Here's how the part is built. I have some questions about the finished solid (model axes, mm). A direction names the side the tool comes from. Round coordinates to 2 decimals unless told otherwise and drop trailing zeros. Write each loop counter-clockwise with the first axis right and the second up, starting at its lowest first coordinate (ties: lowest second). Pieces come first, ordered by that corner, then holes. Notation, with made-up numbers: (-22, 2.5) - (16, 2.5) arc R34 ccw to (16, 36.5) - close; hole circle Ø8 at (-3, -16). An arc over 180 degrees is marked (long way). Write item = value, one per line. Start each with the question number.
Item 1: If we section it at C-C (x = 1.5): Please give me the cut outline in (y, z).
Item 2: If I drill on line 1 along X through (y, z) = (1.25, 1.5); line 2 along X through (y, z) = (0.5, 9), over which ranges is the centre line in solid material (lowest first)? Write a range as [from, to].
Item 3: If we section it at A-A (z = 9.5): Please give me the cut outline in (x, y), and give its area (3 significant figures).
Item 4: Which directions (+Z, -Z, +X, -X, +Y, -Y) give clear straight access to the entire face, cutting with the end or side of a thin tool? Please do faces 1 (the face through (0.2, -2, 9)), 2 (the face through (-0.2, -2, 2)), 3 (the face through (-2, 0.2, 2)).
Item 5: If we section it at B-B (y = -2): Please give me the cut outline in (x, z), and give its area (3 significant figures).
Item 6: For P1, Ø1.8, axis at x = 2, z = 2, coming from the +Y side; P2, Ø1.5, axis at x = 2, y = 1, coming from the -Z side; P3, Ø1.1, axis at y = -3, z = 2, coming from the +X side; P4, Ø0.9, axis at y = 2, z = 10, coming from the -X side, each with a flat end and sliding along its axis, tell me the tip position at first contact or that it passes through.
Item 7: Thinking about a two-plate mould opening in Z: for faces 4 (the face through (0.2, -2, 2)), 5 (the face through (-2.313, 0.003, 14.391)), which applies, pulls with the +Z half, pulls with the -Z half, needs draft (parallel to the pull), parting line crosses it, or undercut?
```python
from build123d import *

# Parameters (mm, degrees)
F3_DEPTH = 0.2
F4_COUNT = 4


# Not quite as in the source:
# - a feature names something its author has since deleted; it is built from what else it names


with BuildPart() as f1:
    # F0 (on Front) → F1 (revolve)
    with BuildSketch(Plane.XZ):
        with BuildLine():
            Line((0, 24.5833333333), (0, 0))
            Line((0, 0), (0.6944444444, 0))
            Line((0.6944444444, 0), (0.6944444444, 0.2777777778))
            Line((0.6944444444, 0.2777777778), (0.9097222222, 0.625))
            Line((0.9097222222, 0.625), (0.9097222222, 20.8333333333))
            ThreePointArc((0.9097222222, 20.8333333333), (0.6790405117, 22.7627175953), (0, 24.5833333333))
        make_face()
    revolve(axis=Axis((0, 0, 12.2916666667), (0, 0, 1)))

    # F2 (on Front) → F3 (join, symmetric)
    with BuildSketch(Plane.XZ):
        with BuildLine():
            Line((0, 0.625), (0, 0.5555555556))
            Line((0, 0.5555555556), (2.7430555556, 0.5555555556))
            Line((2.7430555556, 0.5555555556), (2.7430555556, 1.1111111111))
            Line((2.7430555556, 1.1111111111), (3.8194444444, 1.1111111111))
            Line((3.8194444444, 1.1111111111), (3.3333333333, 2.7777777778))
            Line((3.3333333333, 2.7777777778), (0.8, 2.7777777778))
            Line((0.8, 2.7777777778), (0.8, 2.9458333333))
            Line((0.8, 2.9458333333), (1.1180555556, 3.2638888889))
            Line((1.1180555556, 3.2638888889), (1.1180555556, 4.1666666667))
            Line((1.1180555556, 4.1666666667), (2.7430555556, 4.1666666667))
            Line((2.7430555556, 4.1666666667), (2.7430555556, 12.9166666667))
            ThreePointArc((2.7430555556, 12.9166666667), (2.3012216629, 14.4095607148), (1.1180555556, 15.4215230609))
            Line((1.1180555556, 15.4215230609), (1.1180555556, 18.7331644265))
            Line((1.1180555556, 18.7331644265), (0, 21.8049968191))
            Line((0, 21.8049968191), (0, 0.625))
        make_face()
    extrude(amount=F3_DEPTH, both=True)

    # F4: F1 ×4 about axis
    f4_axis = Axis((0, 0, 0.625), (0, 0, 1))


with BuildPart() as f1_1:
    add(f1.part)
    for i in range(1, F4_COUNT):
        add(f1.part.rotate(f4_axis, i * 360 / F4_COUNT))


solid = f1_1.part
```
Reply:
q1.outline = (-0.2, 0.56) - (0.2, 0.56) - (0.2, 2.78) - (-0.2, 2.78) - close; (-0.2, 4.17) - (0.2, 4.17) - (0.2, 15.21) - (-0.2, 15.21) - close
q2.line_1 = [-0.2, 0.2]
q2.line_2 = [-0.76, 0.76]
q3.outline = (-2.74, -0.2) - (-0.89, -0.2) arc R0.91 ccw to (-0.2, -0.89) - (-0.2, -2.74) - (0.2, -2.74) - (0.2, -0.89) arc R0.91 ccw to (0.89, -0.2) - (2.74, -0.2) - (2.74, 0.2) - (0.89, 0.2) arc R0.91 ccw to (0.2, 0.89) - (0.2, 2.74) - (-0.2, 2.74) - (-0.2, 0.89) arc R0.91 ccw to (-0.89, 0.2) - (-2.74, 0.2) - close
q3.area = 5.55 mm2
q4.face_1 = +Z, -Z, +X, -Y
q4.face_2 = +Z, -Z, -X, -Y
q4.face_3 = +Z, -Z, -X, +Y
q5.outline = (-0.2, 0.56) - (0.2, 0.56) - (0.2, 2.78) - (-0.2, 2.78) - close; (-0.2, 4.17) - (0.2, 4.17) - (0.2, 14.79) - (-0.2, 14.79) - close
q5.area = 5.14 mm2
q6.P1 = 0.2
q6.P2 = through
q6.P3 = 0.2
q6.P4 = -0.2
q7.face_4 = needs draft
q7.face_5 = pulls with the +Z half
